from build123d import *

# Parameters (mm, degrees)
SKETCH1_R           = 1.651
BOSS_EXTRUDE1_DEPTH = 2.3114
SKETCH2_W           = 50.038
SKETCH2_H           = 15.494
BOSS_EXTRUDE2_DEPTH = 13.5128


with BuildPart() as part:
    # Sketch1 → Boss-Extrude1 (new body)
    with BuildSketch(Plane(origin=(0, 0, 0), x_dir=(1, 0, 0), z_dir=(0, 1, 0))):
        Polygon((0, 0), (10.4648, 0), (10.4648, 6.604), (50.038, 6.604), (50.038, 28.702), (39.5732, 28.702), (39.5732, 22.098), (0, 22.098), align=None)
        with Locations(Location((5.2324, 3.683, 0), (0, 0, 270))):
            Circle(SKETCH1_R, mode=Mode.SUBTRACT)
        with Locations(Location((44.8056, 25.019, 0), (0, 0, 270))):
            Circle(SKETCH1_R, mode=Mode.SUBTRACT)
    extrude(amount=BOSS_EXTRUDE1_DEPTH)

    # Sketch2 → Boss-Extrude2 (add)
    with BuildSketch(Plane(origin=(0, 2.3114, 0), x_dir=(1, 0, 0), z_dir=(0, 1, 0))):
        with Locations((25.019, 14.351)):
            Rectangle(SKETCH2_W, SKETCH2_H)
    extrude(amount=BOSS_EXTRUDE2_DEPTH)


solid = part.part
Can you work these out from the model? Positions are in its coordinate system, mm. A direction names the side the tool comes from. Coordinates: 2 decimals unless noted, no trailing zeros. Write each loop counter-clockwise with the first axis right and the second up, starting at its lowest first coordinate (ties: lowest second). Pieces come first, ordered by that corner, then holes. Notation, with made-up numbers: (9, 78.5) -> (23, 78.5) arc R23 ccw to (23, 102.5) -> close; hole circle Ø11 at (2, -27). An arc over 180 degrees is marked (long way). Write each question's results on one line, items separated by ' | '. Start each with the question number.
Item 1: If we section it at D-D, the plane y = 14: Write out the boundary of the cut face in (x, z).
Item 2: On a 3-axis mill with a long thin cutter (end or side, diameter ignored), from which of +Z, -Z, +X, -X, +Y, -Y can I reach the whole of each face in a straight line? I mean faces 5 (the flat face through (0, 8, -13)), 6 (the flat face through (10.465, 1, -3)), 7 (the flat face through (25, 0, -15)), 8 (the flat face through (45, 2.311, -27)), 9 (the flat face through (5.16, 2.311, -1.88)). Say none if no direction works.
Item 3: If we section it at B-B, the plane y = 1: Write out the boundary of the cut face in (x, z).
Item 4: If we section it at A-A, the plane z = -24.5: Write out the boundary of the cut face in (x, y).
Item 5: Please list where these lines run through material, in increasing order: probe 1 along Z at (x, y) = (23, 7.25); probe 2 along Z at (x, y) = (42, 1.75).
Item 6: I'm going to push flat-ended pins straight in: P1, Ø4.5, axis at x = 44.81, z = -25.02, coming from the -Y side; P2, Ø8, axis at x = 35, y = 10.5, coming from the +Z side; P3, Ø6, axis at x = 35.5, y = 6, coming from the -Z side; P4, Ø1.8, axis at y = 0.5, z = -26, coming from the -X side. Where does each tip first touch, or does it pass through?
Item 7: If we section it at C-C, the plane x = 42.5: Write out the boundary of the cut face in (y, z), and give its area (3 significant figures).
Item 8: Thinking about a two-plate mould opening in X: for faces 1 (the flat face through (39.573, 1, -25)), 2 (the cylindrical face through (3.62, 1.14, -4.04)), 3 (the flat face through (5, 1, 0)), 4 (the cylindrical face through (43.2, 1.1, -25.4)), which applies, released by +X, released by -X, zero draft, split by the parting line, or undercut?
Answer block:
1) outline: (0, -22.1) -> (50.04, -22.1) -> (50.04, -6.6) -> (0, -6.6) -> close
2) face 5: +Z, -Z, -X, +Y, -Y | face 6: +Z, +X, +Y, -Y | face 7: +Z, -Z, +X, -X, -Y | face 8: -Z, +X, -X, +Y | face 9: +Z, +X, -X, +Y
3) outline: (0, -22.1) -> (39.57, -22.1) -> (39.57, -28.7) -> (50.04, -28.7) -> (50.04, -6.6) -> (10.46, -6.6) -> (10.46, 0) -> (0, 0) -> close; hole circle Ø3.3 at (5.23, -3.68); hole circle Ø3.3 at (44.81, -25.02)
4) outline: (39.57, 0) -> (43.24, 0) -> (43.24, 2.31) -> (39.57, 2.31) -> close; (46.37, 0) -> (50.04, 0) -> (50.04, 2.31) -> (46.37, 2.31) -> close
5) probe 1: -22.1 to -6.6 | probe 2: -28.7 to -6.6
6) P1: y = 0 | P2: z = -6.6 | P3: z = -22.1 | P4: x = 39.57
7) outline: (0, -28.7) -> (2.31, -28.7) -> (2.31, -22.1) -> (15.82, -22.1) -> (15.82, -6.6) -> (0, -6.6) -> close | area: 260 mm²
8) face 1: released by -X | face 2: undercut | face 3: zero draft | face 4: undercut
